```python
from build123d import *

# Parameters (mm, degrees)
F0_R     = 43.18
F0_R_2   = 3.571875
F1_DEPTH = 4.318


with BuildPart() as f1:
    # F0 (on Front) → F1 (new body)
    with BuildSketch(Plane.XZ):
        Circle(F0_R)
        with BuildLine():
            ThreePointArc((-18.889089, -2.470793), (-25.040397, 0), (-18.889089, 2.470793))
            ThreePointArc((-18.889089, 2.470793), (1.238013, 19.00973), (19.05, 0))
            ThreePointArc((19.05, 0), (1.238013, -19.00973), (-18.889089, -2.470793))
        make_face(mode=Mode.SUBTRACT)
        with Locations((22.86, 0)):
            Circle(F0_R_2, mode=Mode.SUBTRACT)
    extrude(amount=F1_DEPTH)


solid = f1.part
```
Input: part model. Units: mm. Frame: model coordinates. Round coordinates to 2 decimals unless told otherwise and drop trailing zeros. Loops run counter-clockwise (first coordinate to the right, second up) from the corner with the lowest first, then second, coordinate; pieces in that order, holes last. Notation, with made-up numbers: (12, 34) -> (40, 34) arc R14 cw to (40, 45) -> close; hole circle Ø10 at (41.25, -16.5). An arc over 180 degrees is marked (long way). Write each question's results on one line, items separated by ' | '.
1. Section A-A (x = 0). Return loops of the section in (y, z).
Geometry results:
outline: (-4.32, -43.18) -> (0, -43.18) -> (0, -19.05) -> (-4.32, -19.05) -> close; (-4.32, 19.05) -> (0, 19.05) -> (0, 43.18) -> (-4.32, 43.18) -> close
2. Ray query, line 1 (Z direction, x = 22.86, y = -1); line 2 (X direction, y = -1, z = 10.5); line 3 (X direction, y = -0.45, z = -11.5). Return the intervals inside material, ascending. Write a range as from..to.
Geometry results:
line 1: -36.63..-3.57, 3.57..36.63 | line 2: -41.88..-15.9, 15.9..41.88 | line 3: -41.62..-15.19, 15.19..41.62
3. Section C-C (y = -1.85). Return loops of the section in (x, z).
Geometry results:
outline: circle Ø86.36 at (0, 0); hole (-18.89, -2.47) arc R19.05 ccw (long way) to (-18.89, 2.47) arc R3.57 ccw (long way) to start; hole circle Ø7.14 at (22.86, 0)
4. First-contact query: P1, Ø5.5, axis at x = -21.47, z = 0, coming from the +Y side; P2, Ø1, axis at x = -7.5, y = -3.5, coming from the -Z side. Flat tips, straight axial feed; report the tip coordinate or a pass-through.
Geometry results:
P1: through | P2: z = -42.61
5. Section D-D (x = -30). Return loops of the section in (y, z).
Geometry results:
outline: (-4.32, -31.06) -> (0, -31.06) -> (0, 31.06) -> (-4.32, 31.06) -> close
6. Mould query, pull axis Z, two halves, no side actions, for faces 1 (the face through (19, 0, -9)), 2 (the face through (-25.04, -2.13, -0.12)), 3 (the face through (-31.83, -2.13, 29.18)), 4 (the face through (19.29, -2.13, 0.16)). Classes: +Z half, -Z half, draft (parallel to the pull), parting line (faces both ways), or undercut.
Geometry results:
face 1: draft | face 2: undercut | face 3: parting line | face 4: undercut
7. Section B-B (z = -15.5). Return loops of the section in (x, y).
Geometry results:
outline: (-40.3, -4.32) -> (-11.07, -4.32) -> (-11.07, 0) -> (-40.3, 0) -> close; (11.07, -4.32) -> (40.3, -4.32) -> (40.3, 0) -> (11.07, 0) -> close
